Source: CAD feature listing. Evaluate the final solid. Frame: model axes, mm. A direction names the side the tool comes from. Give positions to 0.01 mm unless a question says otherwise; leave off trailing zeros. Order: outer loops, then holes, each group sorted by start corner. A loop starts at its lowest first (then second) coordinate and runs counter-clockwise, first axis right, second up.
1) Material intervals for line 1 (X direction, y = 4.25, z = -0.1); line 2 (Y direction, x = 4.25, z = 0); line 3 (Y direction, x = 3.5, z = -0.05), sorted ascending.
2) Access query for faces 4 (the face through (0.1, 4.5, 0.45)), 5 (the face through (5.106, 2.908, -0.006)), 6 (the face through (-3.85, -4.74, 0.01)). Directions: +Z, -Z, +X, -X, +Y, -Y. A direction counts if a zero-diameter tool reaches every point of the face in a straight line with its end or side. Return the directions, or none.
3) Section C-C, the plane y = 4.25. Return loops of the section in (x, z), plus the area to 3 significant figures.
4) Section A-A, the plane y = -2.5. Return loops of the section in (x, z) (3 decimals), plus the area to 3 significant figures.
5) Draft query along Y for faces 1 (the face through (3.315, -3, 0)), 2 (the face through (5, -1.3, 0)), 3 (the face through (-6, -5.312, 0)). Return one class per face: released by +Y, released by -Y, zero draft, split by the parting line, or undercut.
6) Section B-B, the plane x = 5.5. Return loops of the section in (y, z), plus the area to 3 significant figures.
```python
from build123d import *

# Parameters (mm, degrees)
SKETCH3_W               = 8.375
SKETCH3_H               = 0.9
CUT_EXTRUDE1_DEPTH      = 12.852584106
CUT_EXTRUDE1_DEPTH_BACK = 12.852584106
SKETCH4_OUTSIDE_W       = 23.492
SKETCH4_OUTSIDE_H       = 23.492
FILLET1_R               = 0.63
FILLET2_R               = 0.7875
FILLET3_R               = 1.89
FILLET4_R               = 0.1575


with BuildPart() as part:
    # Sketch3 → Revolve1 (revolve)
    with BuildSketch(Plane(origin=(0, 0, 0), x_dir=(1, 0, 0), z_dir=(0, 1, 0))):
        with Locations((-4.1875, 0)):
            Rectangle(SKETCH3_W, SKETCH3_H)
    revolve(axis=Axis((0, 0, -0.45), (0, 0, 1)))

    # Sketch4 outside → Cut-Extrude1 (cut, two sides: drawn at the far end of the back side and taken through both)
    with BuildSketch(Plane.XY.offset(-CUT_EXTRUDE1_DEPTH_BACK)):
        Rectangle(SKETCH4_OUTSIDE_W, SKETCH4_OUTSIDE_H)
        with BuildLine():
            Line((-3.315, -2.054452482), (-3.315, -5.3125))
            Line((-3.315, -5.3125), (-6.474408757, -5.3125))
            ThreePointArc((-6.474408757, -5.3125), (0, 8.375), (6.474408757, -5.3125))
            Line((6.474408757, -5.3125), (3.315, -5.3125))
            Line((3.315, -5.3125), (3.315, -2.054452482))
            Line((3.315, -2.054452482), (3.315, -1.3))
            Line((3.315, -1.3), (3.676955262, -1.3))
            Line((3.676955262, -1.3), (6.64647189, -1.3))
            ThreePointArc((6.64647189, -1.3), (5.150270007, 2.854307126), (1.381111973, 5.154380056))
            Line((1.381111973, 5.154380056), (1.009394276, 3.767110723))
            ThreePointArc((1.009394276, 3.767110723), (0, 3.9), (-1.009394276, 3.767110723))
            Line((-1.009394276, 3.767110723), (-1.381111973, 5.154380056))
            ThreePointArc((-1.381111973, 5.154380056), (-5.150270007, 2.854307126), (-6.64647189, -1.3))
            Line((-6.64647189, -1.3), (-3.676955262, -1.3))
            Line((-3.676955262, -1.3), (-3.315, -1.3))
            Line((-3.315, -1.3), (-3.315, -2.054452482))
        make_face(mode=Mode.SUBTRACT)
    extrude(amount=CUT_EXTRUDE1_DEPTH + CUT_EXTRUDE1_DEPTH_BACK, mode=Mode.SUBTRACT)

    # Fillet1
    fillet1_edges = [part.edges().sort_by_distance(p)[0] for p in [
        (3.315, -1.3, 0),
        (1.381111973, 5.154380056, 0),
        (-1.381111973, 5.154380056, 0),
        (-3.315, -1.3, 0),
    ]]
    fillet(fillet1_edges, radius=FILLET1_R)

    # Fillet2
    fillet2_edges = [part.edges().sort_by_distance(p)[0] for p in [
        (6.64647189, -1.3, 0),
        (-6.64647189, -1.3, 0),
    ]]
    fillet(fillet2_edges, radius=FILLET2_R)

    # Fillet3
    fillet3_edges = [part.edges().sort_by_distance(p)[0] for p in [
        (3.315, -5.3125, 0),
        (-3.315, -5.3125, 0),
    ]]
    fillet(fillet3_edges, radius=FILLET3_R)

    # Fillet4
    fillet4_edges = [part.edges().sort_by_distance(p)[0] for p in [
        (1.009394276, 3.767110723, 0),
        (-1.009394276, 3.767110723, 0),
    ]]
    fillet(fillet4_edges, radius=FILLET4_R)


solid = part.part
```
From the geometry:
1. line 1: x = -7.22 to -3.58, -1.14 to 1.14, 3.58 to 7.22
1. line 2: y = -5.05 to -1.3, 3.76 to 7.22
1. line 3: y = -4.24 to -1.48, 4.3 to 7.61
2. face 4: +Z, +X, -X, +Y, -Y
2. face 5: +Z, -Z
2. face 6: +Z, -Z, -Y
3. outline: (-7.22, -0.45) - (-3.58, -0.45) - (-3.58, 0.45) - (-7.22, 0.45) - close; (-1.14, -0.45) - (1.14, -0.45) - (1.14, 0.45) - (-1.14, 0.45) - close; (3.58, -0.45) - (7.22, -0.45) - (7.22, 0.45) - (3.58, 0.45) - close
3. area: 8.59 mm2
4. outline: (-7.993, -0.45) - (-3.315, -0.45) - (-3.315, 0.45) - (-7.993, 0.45) - close; (3.315, -0.45) - (7.993, -0.45) - (7.993, 0.45) - (3.315, 0.45) - close
4. area: 8.42 mm2
5. face 1: zero draft
5. face 2: undercut
5. face 3: released by -Y
6. outline: (-5.31, -0.45) - (-1.3, -0.45) - (-1.3, 0.45) - (-5.31, 0.45) - close; (2.38, -0.45) - (6.32, -0.45) - (6.32, 0.45) - (2.38, 0.45) - close
6. area: 7.15 mm2
